from build123d import *

# Parameters (mm, degrees)
EXTRUDE_THIN6_START      = -10
SKETCH10_R               = 10
SKETCH10_R_2             = 5
EXTRUDE_THIN6_DEPTH      = 40
BOSS_EXTRUDE3_REACH      = 42.311
BOSS_EXTRUDE3_END_RADIUS = 10
SKETCH11_R               = 4
SKETCH12_W               = 4.268669827
SKETCH12_H               = 50.716029666
CUT_EXTRUDE2_DEPTH       = 4
BOSS_EXTRUDE4_START      = -20
SKETCH13_W               = 8
SKETCH13_H               = 6
BOSS_EXTRUDE4_DEPTH      = 24
FILLET3_R                = 4
FILLET4_R                = 2


with BuildPart() as part:
    # Sketch10 → Extrude-Thin6 (new body)
    with BuildSketch(Plane(origin=(0, 0, 0), x_dir=(-1, 0, 0), z_dir=(0, 0, -1)).offset(EXTRUDE_THIN6_START)):
        Circle(SKETCH10_R)
        Circle(SKETCH10_R_2, mode=Mode.SUBTRACT)
    extrude(amount=EXTRUDE_THIN6_DEPTH)

    # Boss-Extrude3: up to this cylinder (the profile starts outside it)
    boss_extrude3_end = Plane(origin=(0, 0, -15), z_dir=(0, 0, 1)) * Cylinder(BOSS_EXTRUDE3_END_RADIUS, 105.622, mode=Mode.PRIVATE)
    # Sketch11 → Boss-Extrude3 (add, up to the surface)
    with BuildSketch(Plane(origin=(0, 15, 0), x_dir=(1, 0, 0), z_dir=(0, 1, 0)), mode=Mode.PRIVATE) as boss_extrude3_sk1:
        with Locations(Location((0, 15, 0), (0, 0, 270))):
            Circle(SKETCH11_R)
    boss_extrude3_tool1 = extrude(boss_extrude3_sk1.sketch, amount=-BOSS_EXTRUDE3_REACH, mode=Mode.PRIVATE) - boss_extrude3_end
    add(boss_extrude3_tool1.solids().sort_by_distance((0, 15, -15))[0])

    # Sketch12 → Cut-Extrude2 (cut)
    with BuildSketch(Plane(origin=(0, 15, 0), x_dir=(1, 0, 0), z_dir=(0, 1, 0))):
        with Locations((-1.865665086, 44.348981699)):
            Rectangle(SKETCH12_W, SKETCH12_H)
    extrude(amount=-CUT_EXTRUDE2_DEPTH, mode=Mode.SUBTRACT)

    # Sketch13 → Boss-Extrude4 (add)
    with BuildSketch(Plane(origin=(0, 0, -18.990966866), x_dir=(-1, 0, 0), z_dir=(0, 0, -1)).offset(BOSS_EXTRUDE4_START)):
        with Locations((0, 14)):
            Rectangle(SKETCH13_W, SKETCH13_H)
    extrude(amount=BOSS_EXTRUDE4_DEPTH)

    # Fillet3
    fillet3_edges = [part.edges().sort_by_distance(p)[0] for p in [
        (4, 14, -22.990966866),
        (-4, 14, 1.009033134),
        (4, 14, 1.009033134),
        (-4, 14, -22.990966866),
    ]]
    fillet(fillet3_edges, radius=FILLET3_R - 0.0001)  # a hair under: the kernel refuses the full size

    # Fillet4
    fillet4_edges = [part.edges().sort_by_distance(p)[0] for p in [
        (-4, 17, -10.990966866),
        (4, 17, -10.990966866),
        (2.828456414, 17, -21.81942328),
        (-2.828456414, 17, -21.81942328),
        (2.828456414, 17, -0.162510452),
        (-2.828456414, 17, -0.162510452),
    ]]
    fillet(fillet4_edges, radius=FILLET4_R - 0.0001)  # a hair under: the kernel refuses the full size


solid = part.part
For this review, take the finished solid that the model builds, in its own axes (mm). A direction names the side the tool comes from. Round coordinates to 2 decimals unless told otherwise and drop trailing zeros. Loops run counter-clockwise (first coordinate to the right, second up) from the corner with the lowest first, then second, coordinate; pieces in that order, holes last. Notation, with made-up numbers: (56.25, -24) - (103.25, -24) arc R12 cw to (103.25, -3) - close; hole circle Ø1 at (30, 66.5). An arc over 180 degrees is marked (long way). Use one line per item in the form item = value.
1) Wall thickness on probe 1 along Y at (x, z) = (0, -15.5); probe 2 along Y at (x, z) = (0.25, -21.5); probe 3 along Y at (x, z) = (-2, -1.5): over which ranges is each line inside the solid? List them lowest first.
Solutions:
probe_1 = -10 to -5, 5 to 17
probe_2 = -10 to -4.99, 4.99 to 10, 11 to 16.93
probe_3 = -9.8 to -4.58, 4.58 to 9.8, 11 to 16.94
2) We need section B-B on y = 0. Write out the cut boundary in (x, z).
Solutions:
outline = (-10, -30) - (-5, -30) - (-5, 10) - (-10, 10) - close; (5, -30) - (10, -30) - (10, 10) - (5, 10) - close
3) We need section A-A on z = -5.5. Write out the cut boundary in (x, y).
Solutions:
outline = circle Ø20 at (0, 0); (-4, 11) - (4, 11) - (4, 15) arc R2 ccw to (2, 17) - (-2, 17) arc R2 ccw to (-4, 15) - close; hole circle Ø10 at (0, 0)
4) Tool access review of faces 1 (the face through (-2.859, 13.028, -0.194)), 2 (the face through (3.373, 10.299, -12.85)), 3 (the face through (2.86, 13.03, -21.79)), 4 (the face through (-2.8, 13.03, -21.85)): name each direction out of +Z, -Z, +X, -X, +Y, -Y from which nothing blocks a thin tool from reaching the whole face with its end or side.
Solutions:
face_1 = +Z, -X, +Y
face_2 = none
face_3 = -Z, +X, +Y
face_4 = -Z, -X, +Y
5) Clearance check with flat-ended pins moving along their axes: P1, Ø8, axis at x = -6.5, z = -15, coming from the -Y side; P2, Ø5, axis at x = -7.5, z = 3.5, coming from the -Y side; P3, Ø1, axis at x = -6, z = -11, coming from the -Y side. State where each tip first meets the part, or that it passes through.
Solutions:
P1 = -9.68
P2 = -8.66
P3 = -8.35
6) We need section D-D on z = -23.5. Write out the cut boundary in (x, y), then the cut area to 3 significant figures.
Solutions:
outline = circle Ø20 at (0, 0); hole circle Ø10 at (0, 0)
area = 236 mm2
7) Mouldability with a two-part tool opening along Y and no side actions: class faces 5 (the face through (0, 11, -5)), 6 (the face through (5, -2, 10)), 7 (the face through (-3.4, 16.43, -11.1)) as pulls with the +Y half, pulls with the -Y half, needs draft (parallel to the pull), parting line crosses it, or undercut.
Solutions:
face_5 = undercut
face_6 = needs draft
face_7 = pulls with the +Y half
